Geometry check sheet. Reference: the model listing, model coordinates, mm. Give positions to 0.01 mm unless a question says otherwise; leave off trailing zeros. Write each loop counter-clockwise with the first axis right and the second up, starting at its lowest first coordinate (ties: lowest second). Pieces come first, ordered by that corner, then holes. Notation, with made-up numbers: (-2.5, -4.5) -> (50.5, -4.5) arc R33 cw to (50.5, 29.5) -> close; hole circle Ø7 at (-30, -28). An arc over 180 degrees is marked (long way). One line per item, written item: value.
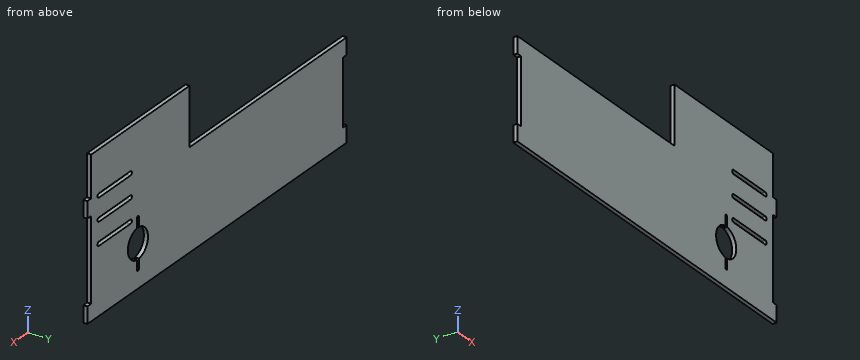
Autodesk Inventor part; units mm, degrees
ref_plane "YZ Plane" through (0, 0, 0) normal (1, 0, 0) x (0, 1, 0)
ref_plane "XZ Plane" through (0, 0, 0) normal (0, 1, 0) x (-1, 0, 0)
ref_plane "XY Plane" through (0, 0, 0) normal (0, 0, 1) x (1, 0, 0)
sketch "Sketch1" plane through (0, 0, 0) normal (0, 1, 0) x (-1, 0, 0)
  line L0 (0, 0) -> (271, 0)
  line L1 (271, 0) -> (271, 84)
  line L2 (271, 84) -> (0, 84)
  line L3 (0, 84) -> (0, 0)
  line L4 (135.5, 84) -> (135.5, 0) construction
  line L5 (0, 84) -> (-4, 84)
  line L6 (-4, 84) -> (-4, 72)
  line L7 (-4, 72) -> (0, 72)
  line L8 (0, 72) -> (0, 84)
  line L9 (0, 0) -> (-4, 0)
  line L10 (-4, 0) -> (-4, 12)
  line L11 (-4, 12) -> (0, 12)
  line L12 (0, 12) -> (0, 0)
  line L13 (271, 84) -> (271, 0)
  line L14 (275, 72) -> (275, 60)
  line L15 (275, 60) -> (271, 60)
  line L16 (271, 60) -> (271, 84)
  line L17 (271, 0) -> (275, 0)
  line L18 (275, 0) -> (275, 12)
  line L19 (275, 12) -> (271, 12)
  line L20 (271, 12) -> (271, 0)
  arc A0 (51.367, 20.056) -> (49.367, 20.056) centre (50.367, 20.056) ccw
  arc A1 (49.367, 41.706) -> (51.367, 41.706) centre (50.367, 41.706) ccw
  line L21 (49.367, 48.706) -> (49.367, 41.706)
  line L22 (50.367, 41.706) -> (50.367, 48.706) construction
  line L23 (51.367, 41.706) -> (51.367, 48.706)
  arc A2 (51.367, 48.706) -> (49.367, 48.706) centre (50.367, 48.706) ccw
  circle A3 centre (50.367, 30.881) radius 10.825
  arc A4 (49.367, 13.056) -> (51.367, 13.056) centre (50.367, 13.056) ccw
  line L24 (49.367, 20.056) -> (49.367, 13.056)
  line L25 (50.367, 20.056) -> (50.367, 13.056) construction
  line L26 (51.367, 13.056) -> (51.367, 20.056)
  line L27 (275, 72) -> (271, 72)
  point P0 (50.367, 45.206)
  point P1 (50.367, 16.556)
  dimension "d0" = 271
  dimension "d2" = 4
  dimension "d3" = 12
  dimension "d4" = 4
  dimension "d5" = 12
  dimension "d20" = 21.65
  dimension "d21" = 7
  dimension "d22" = 2
  dimension "d23" = 7
  dimension "d24" = 2
  dimension "d56" = 50.367
  dimension "d57" = 30.881
  dimension "d58" = 48
  dimension "d59" = 12
  dimension "d60" = 12
extrude "Extrusion1" add sketch "Sketch1" along normal blind 3
sketch "Sketch3" plane through (0, 0, 0) normal (0, -1, 0) x (1, 0, 0)
  line L0 (4, 0) -> (-275, 0)
  line L1 (-270, 114) -> (0, 114)
  line L2 (0, 114) -> (0, 84)
  line L3 (0, 84) -> (-270, 84)
  line L4 (-270, 84) -> (-270, 114)
  line L5 (-275, 84) -> (4, 84)
  point P0 (0, 0)
  point P1 (-275, 72)
  point P2 (4, 84)
  dimension "d28" = 30
extrude "Extrusion2" add sketch "Sketch3" against normal blind 3
sketch "Sketch2" plane through (0, 0, 0) normal (0, -1, 0) x (1, 0, 0)
  circle A0 centre (-25.367, 65.881) radius 1.5 construction
  arc A1 (-49.3681, 20.1022) -> (-49.3681, 41.6598) centre (-50.367, 30.881) ccw construction
  line L0 (-8.367, 65.881) -> (-42.367, 65.881) construction
  line L1 (-8.367, 67.381) -> (-42.367, 67.381)
  line L2 (-42.367, 64.381) -> (-8.367, 64.381)
  arc A2 (-8.367, 64.381) -> (-8.367, 67.381) centre (-8.367, 65.881) ccw
  arc A3 (-42.367, 67.381) -> (-42.367, 64.381) centre (-42.367, 65.881) ccw
  line L3 (-8.367, 82.381) -> (-42.367, 82.381) construction
  line L4 (-8.367, 83.881) -> (-42.367, 83.881)
  line L5 (-42.367, 80.881) -> (-8.367, 80.881)
  arc A4 (-8.367, 80.881) -> (-8.367, 83.881) centre (-8.367, 82.381) ccw
  arc A5 (-42.367, 83.881) -> (-42.367, 80.881) centre (-42.367, 82.381) ccw
  line L6 (-8.367, 49.381) -> (-42.367, 49.381) construction
  line L7 (-8.367, 50.881) -> (-42.367, 50.881)
  line L8 (-42.367, 47.881) -> (-8.367, 47.881)
  arc A6 (-8.367, 47.881) -> (-8.367, 50.881) centre (-8.367, 49.381) ccw
  arc A7 (-42.367, 50.881) -> (-42.367, 47.881) centre (-42.367, 49.381) ccw
  line L9 (-42.367, 65.881) -> (-42.367, 49.381) construction
  line L10 (-42.367, 82.381) -> (-42.367, 65.881) construction
  point P0 (0, 0)
  point P1 (-25.367, 82.381)
  point P2 (-25.367, 49.381)
  dimension "d41" = 3
  dimension "d43" = 25
  dimension "d44" = 35
  dimension "d45" = 17
  dimension "d46" = 3
  dimension "d47" = 17
  dimension "d48" = 3
  dimension "d52" = 17
  dimension "d53" = 3
  dimension "d54" = 16.5
  dimension "d55" = 16.5
extrude "Extrusion3" cut sketch "Sketch2" against normal blind 3
sketch "Sketch4" plane through (0, 0, 0) normal (0, -1, 0) x (1, 0, 0)
  line L0 (-275, 72) -> (-271, 72)
  line L1 (-270, 114) -> (0, 114)
  line L2 (-271, 72) -> (-106, 72)
  line L3 (-106, 72) -> (-106, 114)
  line L4 (-106, 114) -> (-271, 114)
  line L5 (-271, 114) -> (-271, 72)
  point P0 (0, 0)
  dimension "d61" = 165
extrude "Extrusion4" cut sketch "Sketch4" along normal through all both and the other way through all
equation "\"d4\" = d2"
equation "\"d41\" = d40"
equation "\"d45\" = d52"
properties part number "flipper-support2"
1) Sectioned sample at B-B on z = 32. Record the cut outline in (x, y), plus the area to 3 significant figures.
Verdict:
outline: (-271, 0) -> (-61.13, 0) -> (-61.13, 3) -> (-271, 3) -> close; (-39.6, 0) -> (0, 0) -> (0, 3) -> (-39.6, 3) -> close
area: 748 mm^2
2) Sectioned sample at A-A on x = -27.5. Record the cut outline in (y, z), plus the area to 3 significant figures.
Verdict:
outline: (0, 0) -> (3, 0) -> (3, 47.88) -> (0, 47.88) -> close; (0, 50.88) -> (3, 50.88) -> (3, 64.38) -> (0, 64.38) -> close; (0, 67.38) -> (3, 67.38) -> (3, 80.88) -> (0, 80.88) -> close; (0, 83.88) -> (3, 83.88) -> (3, 114) -> (0, 114) -> close
area: 315 mm^2
3) Sectioned sample at D-D on z = 94.5. Record the cut outline in (x, y), plus the area to 3 significant figures.
Verdict:
outline: (-106, 0) -> (0, 0) -> (0, 3) -> (-106, 3) -> close
area: 318 mm^2
4) Depth check by flat-ended pin: pin 1 Ø1.5 at (x, y) = (-273, 2) entering from +Z; pin 2 Ø0.9 at (y, z) = (1, 27) entering from -X; pin 3 Ø0.9 at (y, z) = (1, 16.5) entering from +X. Enter the tip coordinate at first touch or a pass-through.
Verdict:
pin 1: z = 72
pin 2: x = -271
pin 3: x = 0
5) Scan lines: probe 1 along Z at (x, y) = (-8, 1.4); probe 2 along Z at (x, y) = (-123, 1.6); probe 3 along X at (y, z) = (0.3, 54). Record each from-to range of solid material in increasing order.
Verdict:
probe 1: 0 to 47.93, 50.84 to 64.43, 67.34 to 80.93, 83.84 to 114
probe 2: 0 to 72
probe 3: -271 to 0
6) Sectioned sample at C-C on y = 1.9. Give the number of separate pieces and of enclosed holes in the cut face, plus the area to 3 significant figures.
Verdict:
separate pieces: 1
enclosed holes: 4
area: 23,400 mm^2
